Here's how the part is built. I have some questions about the finished solid (model axes, mm). Face numbers are marked on the shaded views. A direction names the side the tool comes from. Give positions to 0.01 mm unless a question says otherwise; leave off trailing zeros. Write each loop counter-clockwise with the first axis right and the second up, starting at its lowest first coordinate (ties: lowest second). Pieces come first, ordered by that corner, then holes. Notation, with made-up numbers: M -17.5,71 L 15.5,71 A4 cw 15.5,77 Z; hole C 34.25,14 d9. An arc over 180 degrees is marked long. Answer as CSV lines item,"result". Start each with the question number.
Q1. Suppose I cut it at B-B (x = 0). Write out the boundary of the cut face in (y, z).
Q2. For pin 1 (1 mm diameter, centred on x = -2.5, z = 71, fed in from +Y); pin 2 (1 mm diameter, centred on y = -33.5, z = 80, fed in from -X); pin 3 (3 mm diameter, centred on x = 4.5, y = -8, fed in from +Z), each with a flat end and sliding along its axis, tell me the tip position at first contact or that it passes through.
Q3. If I drill on line 1 along X through (y, z) = (-4, 78.5); line 2 along Y through (x, z) = (0, 79); line 3 along Y through (x, z) = (0, 34), over which ranges is the centre line in solid material (lowest first)?
Q4. Suppose I cut it at A-A (z = 28.5). Write out the boundary of the cut face in (x, y), then the cut area to 3 significant figures.
Q5. On a 3-axis mill with a long thin cutter (end or side, diameter ignored), from which of +Z, -Z, +X, -X, +Y, -Y can I reach the whole of each face in a straight line? I mean the marked faces 4 and 5. Say none if no direction works.
Q6. Thinking about a two-plate mould opening in X: for the marked faces 1, 2 and 3, which applies, +X half, -X half, draft (parallel to the pull), parting line (faces both ways), or undercut?
```python
from build123d import *

# Parameters (mm, degrees)
F2_R     = 26.8
F0_R     = 85
F4_R     = 25
F5_DEPTH = 158.2
F6_T     = -1.8


with BuildPart() as f3:
    # F2 (on offset) → F3 section 0
    with BuildSketch(Plane.XY.offset(160)):
        Circle(F2_R)
    # F0 (on Top) → F3 section 1
    with BuildSketch(Plane.XY):
        Circle(F0_R)
    loft()

    # F4 (on offset) → F5 (cut)
    with BuildSketch(Plane.XY.offset(160)):
        Circle(F4_R)
    extrude(amount=-F5_DEPTH, mode=Mode.SUBTRACT)

    # F6
    f6_openings = [f3.faces().sort_by_distance(p)[0] for p in [
        (0, 0, 0),
    ]]
    offset(amount=F6_T, openings=f6_openings, kind=Kind.INTERSECTION)


solid = f3.part
```
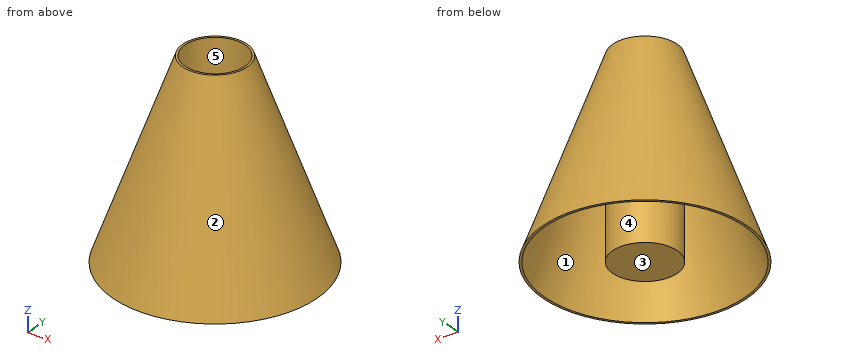
Resolved:
1,outline,"M -85,0 L -83.08,0 L -26.8,154.73 L -26.8,0 L 26.8,0 L 26.8,154.73 L 83.08,0 L 85,0 L 26.8,160 L 25,160 L 25,1.8 L -25,1.8 L -25,160 L -26.8,160 Z"
2,pin 1,"y = 59.3"
2,pin 2,"x = -45.18"
2,pin 3,"z = 1.8"
3,line 1,"-56.3 to -54.38, -26.5 to -24.68, 24.68 to 26.5, 54.38 to 56.3"
3,line 2,"-56.26 to -54.35, -26.8 to -25, 25 to 26.8, 54.35 to 56.26"
3,line 3,"-72.63 to -70.72, -26.8 to -25, 25 to 26.8, 70.72 to 72.63"
4,outline,"C 0,0 d149.27; C 0,0 d53.6; hole C 0,0 d145.44; hole C 0,0 d50"
4,area,"1,180 mm^2"
5,face 4,"-Z"
5,face 5,"+Z"
6,face 1,"undercut"
6,face 2,"parting line"
6,face 3,"draft"
